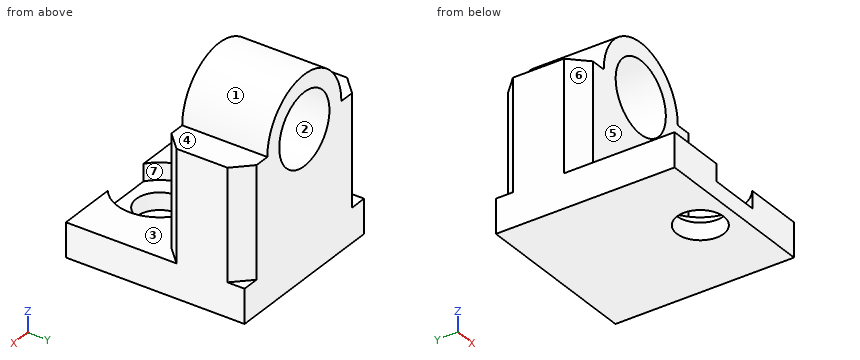
```python
from build123d import *

# Parameters (mm, degrees)
SKETCH_1_W          = 20
SKETCH_1_H          = 32
SKETCH_1_R          = 2.75
EXTRUDE_1_DEPTH     = 4
SKETCH_2_W          = 20
SKETCH_2_H          = 10
EXTRUDE_2_DEPTH     = 13
SKETCH_4_R          = 6.2
EXTRUDE_3_DEPTH     = 10
SKETCH_5_R          = 4.2
CUT_EXTRUDE_1_DEPTH = 13
CHAMFER_1_SIZE      = 2
SKETCH_6_R          = 5
CUT_EXTRUDE_2_DEPTH = 2
SKETCH_7_W          = 20
SKETCH_7_H          = 11
CUT_EXTRUDE_3_DEPTH = 43.339579592


with BuildPart() as part:
    # 草图1 → 凸台-拉伸1 (new body)
    with BuildSketch(Plane.XY):
        with Locations((10, -16)):
            Rectangle(SKETCH_1_W, SKETCH_1_H)
        with Locations((10, -4)):
            Circle(SKETCH_1_R, mode=Mode.SUBTRACT)
        with Locations((10, -28)):
            Circle(SKETCH_1_R, mode=Mode.SUBTRACT)
    extrude(amount=EXTRUDE_1_DEPTH)

    # 草图2 → 凸台-拉伸2 (add)
    with BuildSketch(Plane.XY.offset(4)):
        with Locations((10, -16)):
            Rectangle(SKETCH_2_W, SKETCH_2_H)
    extrude(amount=EXTRUDE_2_DEPTH)

    # 草图4 → 凸台-拉伸3 (add)
    with BuildSketch(Plane.XZ.offset(21)):
        with Locations((10, 17)):
            Circle(SKETCH_4_R)
    extrude(amount=-EXTRUDE_3_DEPTH)

    # 草图5 → 切除-拉伸1 (cut)
    with BuildSketch(Plane(origin=(0, -11, 0), x_dir=(1, 0, 0), z_dir=(0, 1, 0))):
        with Locations(Location((10, -17, 0), (0, 0, 270))):
            Circle(SKETCH_5_R)
    extrude(amount=-CUT_EXTRUDE_1_DEPTH, mode=Mode.SUBTRACT)

    # 倒角1
    chamfer_1_edges = [part.edges().sort_by_distance(p)[0] for p in [
        (0, -11, 10.5),
        (0, -21, 10.5),
        (20, -21, 10.5),
        (20, -11, 10.5),
    ]]
    chamfer(chamfer_1_edges, length=CHAMFER_1_SIZE)

    # 草图6 → 切除-拉伸2 (cut)
    with BuildSketch(Plane.XY.offset(4)):
        with Locations((10, -28)):
            Circle(SKETCH_6_R)
        with Locations((10, -4)):
            Circle(SKETCH_6_R)
    extrude(amount=-CUT_EXTRUDE_2_DEPTH, mode=Mode.SUBTRACT)

    # 草图7 → 切除-拉伸3 (cut, through all)
    with BuildSketch(Plane.XY.offset(4)):
        with Locations((10, -5.5)):
            Rectangle(SKETCH_7_W, SKETCH_7_H)
    extrude(amount=-CUT_EXTRUDE_3_DEPTH, mode=Mode.SUBTRACT)


solid = part.part
```
Input: part model. Units: mm. Frame: model coordinates. Face numbers are marked on the shaded views. A direction names the side the tool comes from. Coordinates: 2 decimals unless noted, no trailing zeros. Loops run counter-clockwise (first coordinate to the right, second up) from the corner with the lowest first, then second, coordinate; pieces in that order, holes last. Notation, with made-up numbers: M -40,67 L -27,67 A22 ccw -27,95 Z; hole C 6,-34 d4. An arc over 180 degrees is marked long. Use a Markdown table: item, result. Add a question column.
1) Section D-D, the plane z = 14. Return the cut outline in (x, y), plus the area to 3 significant figures.
2) Pin query (flat end, axial travel): P1, Ø1.5, axis at y = -17, z = 19.5, coming from the +X side; P2, Ø1.1, axis at x = 2.5, y = -17, coming from the +Z side; P3, Ø7.5, axis at x = 10, z = 17, coming from the -Y side; P4, Ø8, axis at x = 10, y = -28, coming from the +Z side. Return the tip coordinate at first contact, or that it passes through.
3) Section B-B, the plane y = -28. Return the cut outline in (x, z), plus the area to 3 significant figures.
4) Section C-C, the plane y = -16. Return the cut outline in (x, z).
5) Section A-A, the plane x = 10. Return the cut outline in (y, z).
6) Line query: L1, parallel to X at y = -28, z = 1.5; L2, parallel to Y at x = 10, z = 0.85; L3, parallel to Y at x = 12.5, z = 21. Output: solid intervals per line, ascending. Write a range as from..to.
7) Draft query along X for the marked faces 1, 2 and 3. Return one class per face: +X half, -X half, draft (parallel to the pull), parting line (faces both ways), or undercut.
8) Set-up query: the marked faces 4, 5, 6 and 7. Return all of +Z, -Z, +X, -X, +Y, -Y with unobstructed straight access to the full face (end or side cutting, diameter ignored); none if empty.
Answer below:
| question | item | result |
|---|---|---|
| 1 | outline | M 0,-19 L 2,-21 L 7.06,-21 L 7.06,-11 L 2,-11 L 0,-13 Z; M 12.94,-21 L 18,-21 L 20,-19 L 20,-13 L 18,-11 L 12.94,-11 Z |
| 1 | area | 133 mm2 |
| 2 | P1 | x = 15.95 |
| 2 | P2 | z = 17 |
| 2 | P3 | through |
| 2 | P4 | z = 2 |
| 3 | outline | M 0,0 L 7.25,0 L 7.25,2 L 5,2 L 5,4 L 0,4 Z; M 12.75,0 L 20,0 L 20,4 L 15,4 L 15,2 L 12.75,2 Z |
| 3 | area | 49.0 mm2 |
| 4 | outline | M 0,0 L 20,0 L 20,17 L 16.2,17 A6.2 ccw 3.8,17 L 0,17 Z; hole C 10,17 d8.4 |
| 5 | outline | M -32,0 L -30.75,0 L -30.75,2 L -32,2 Z; M -25.25,0 L -11,0 L -11,12.8 L -21,12.8 L -21,4 L -23,4 L -23,2 L -25.25,2 Z; M -21,21.2 L -11,21.2 L -11,23.2 L -21,23.2 Z |
| 6 | L1 | 0..7.25, 12.75..20 |
| 6 | L2 | -32..-30.75, -25.25..-11 |
| 6 | L3 | -21..-11 |
| 7 | face 1 | parting line |
| 7 | face 2 | undercut |
| 7 | face 3 | draft |
| 8 | face 4 | +Z, +X, +Y, -Y |
| 8 | face 5 | +Z, +X, -X, -Y |
| 8 | face 6 | +Z, -X, -Y |
| 8 | face 7 | +Z |
